Autodesk Inventor part; units mm, degrees
ref_plane "YZ Plane" through (0, 0, 0) normal (1, 0, 0) x (0, 1, 0)
ref_plane "XZ Plane" through (0, 0, 0) normal (0, 1, 0) x (-1, 0, 0)
ref_plane "XY Plane" through (0, 0, 0) normal (0, 0, 1) x (1, 0, 0)
sketch "Sketch1" plane through (0, 0, 0) normal (0, 0, 1) x (1, 0, 0)
  circle A0 centre (0, 0) radius 7.62
  circle A1 centre (0, -40.005) radius 30.48
  circle A2 centre (0, 0) radius 1.55
  circle A3 centre (0, -40.005) radius 1.55
  line L0 (-25.4, 14.478) -> (25.4, 14.478)
  line L1 (25.4, 14.478) -> (25.4, -87.122)
  line L2 (25.4, -87.122) -> (-25.4, -87.122)
  line L3 (-25.4, -87.122) -> (-25.4, 14.478)
  line L4 (-25.4, -87.122) -> (-38.1, -87.122)
  line L5 (-38.1, -87.122) -> (-38.1, -78.232)
  line L6 (-38.1, -78.232) -> (-25.4, -78.232)
  line L7 (25.4, -87.122) -> (38.1, -87.122)
  line L8 (38.1, -87.122) -> (38.1, -78.232)
  line L9 (38.1, -78.232) -> (25.4, -78.232)
  dimension "d0" = 40.005
  dimension "d1" = 15.24
  dimension "d2" = 60.96
  dimension "d3" = 3.1
  dimension "d4" = 3.1
  dimension "d5" = 14.478
  dimension "d6" = 25.4
  dimension "d7" = 25.4
  dimension "d8" = 101.6
  dimension "d9" = 12.7
  dimension "d10" = 12.7
  dimension "d11" = 8.89
extrude "Extrusion1" add sketch "Sketch1" along normal blind 12.7 contours A0 | L1 A1 L3 | A1 L3 L0 L1 | L1 L2 L3 A1 | L9 L8 L7 L1 | L3 L4 L5 L6
sketch "Sketch3" plane through (0, 0, 12.7) normal (0, 0, 1) x (1, 0, 0)
  line L0 (-25.4, -78.232) -> (-38.1, -78.232)
  line L1 (38.1, -87.122) -> (38.1, -78.232)
  line L2 (-38.1, -78.232) -> (38.1, -78.232)
  line L3 (38.1, -78.232) -> (38.1, -87.122)
  line L4 (38.1, -87.122) -> (-38.1, -87.122)
  line L5 (-38.1, -87.122) -> (-38.1, -78.232)
  point P0 (0, 0)
extrude "Extrusion3" add sketch "Sketch3" along normal blind 12.7
sketch "Sketch5" plane through (0, 0, 0) normal (0, 0, -1) x (-1, 0, 0)
  line L0 (38.1, -87.122) -> (-38.1, -87.122)
  line L1 (38.1, -78.232) -> (38.1, -87.122)
  line L2 (-38.1, -87.122) -> (38.1, -87.122)
  line L3 (38.1, -87.122) -> (38.1, -78.232)
  line L4 (38.1, -78.232) -> (-38.1, -78.232)
  line L5 (-38.1, -78.232) -> (-38.1, -87.122)
  point P0 (0, 0)
extrude "Extrusion4" add sketch "Sketch5" along normal blind 4.9022
properties part number "Frame"
For this review, take the finished solid that the model builds, in its own axes (mm). A direction names the side the tool comes from. Give positions to 0.01 mm unless a question says otherwise; leave off trailing zeros. Write each loop counter-clockwise with the first axis right and the second up, starting at its lowest first coordinate (ties: lowest second). Pieces come first, ordered by that corner, then holes. Notation, with made-up numbers: M -22.75,51.5 L 24.25,51.5 A20 ccw 24.25,75.5 Z; hole C 89,-14.75 d11. An arc over 180 degrees is marked long. Answer as a JSON object with one key per item and string values. Group by question number.
Item 1: Tool access review of faces 1 (the flat face through (0, -31, 0)), 2 (the flat face through (0, -31, 12.7)), 3 (the flat face through (-1, -83, 25.4)), 4 (the flat face through (25.4, -31, 6)), 5 (the flat face through (38.1, -83, 10)): name each direction out of +Z, -Z, +X, -X, +Y, -Y from which nothing blocks a thin tool from reaching the whole face with its end or side.
Item 2: For pin 1 Ø10 at (y, z) = (-21.5, 9.5) entering from -X; pin 2 Ø6.5 at (y, z) = (-16, 4) entering from +X; pin 3 Ø1 at (x, y) = (7, -64) entering from +Z; pin 4 Ø2 at (y, z) = (-31.5, 14.5) entering from +X, all flat-tipped, find the tip position at first contact; note any pin that passes through.
Item 3: For probe 1 along Y at (x, z) = (0, 7) (3 decimals); probe 2 along Z at (x, y) = (13, -13.5); probe 3 along X at (y, z) = (-20, 12), list the stretches that pass through material, from the lowest coordinate up. Write a range as [from, to].
Item 4: Consider section B-B on x = 0. Write out the cut boundary in (y, z) (3 decimals).
Item 5: Draft analysis for pull direction X (two halves, no side actions). For faces 6 (the cylindrical face through (-0.336, -38.492, 6.261)), 7 (the cylindrical face through (0.715, 1.375, 6.261)), 8 (the flat face through (-1, -78.232, 14)), 9 (the flat face through (-25.4, -33, 6)), state which applies: +X half, -X half, draft (parallel to the pull), parting line (faces both ways), or undercut.
Item 6: Consider section D-D on x = -28. Write out the cut boundary in (y, z), plus the area to 3 significant figures.
Item 7: Consider section A-A on y = 0. Write out the cut boundary in (x, z).
Item 8: Consider section C-C on z = 6.5. Write out the cut boundary in (x, y) (3 decimals).
Check result:
{
 "1": {"face 1": "-Z, +X, -X, +Y", "face 2": "+Z, +X, -X, +Y", "face 3": "+Z, +X, -X, +Y, -Y", "face 4": "+Z, -Z, +X, +Y", "face 5": "+Z, -Z, +X, +Y, -Y"},
 "2": {"pin 1": "stops at x = -25.4", "pin 2": "stops at x = 25.4", "pin 3": "stops at z = 12.7", "pin 4": "passes through"},
 "3": {"probe 1": "y = [-87.122, -41.555], [-38.455, -1.55], [1.55, 14.478]", "probe 2": "z = [0, 12.7]", "probe 3": "x = [-25.4, 25.4]"},
 "4": {"outline": "M -87.122,-4.902 L -78.232,-4.902 L -78.232,0 L -41.555,0 L -41.555,12.7 L -78.232,12.7 L -78.232,25.4 L -87.122,25.4 Z; M -38.455,0 L -1.55,0 L -1.55,12.7 L -38.455,12.7 Z; M 1.55,0 L 14.478,0 L 14.478,12.7 L 1.55,12.7 Z"},
 "5": {"face 6": "undercut", "face 7": "undercut", "face 8": "draft", "face 9": "-X half"},
 "6": {"outline": "M -87.12,-4.9 L -78.23,-4.9 L -78.23,25.4 L -87.12,25.4 Z", "area": "269 mm^2"},
 "7": {"outline": "M -25.4,0 L -1.55,0 L -1.55,12.7 L -25.4,12.7 Z; M 1.55,0 L 25.4,0 L 25.4,12.7 L 1.55,12.7 Z"},
 "8": {"outline": "M -38.1,-87.122 L 38.1,-87.122 L 38.1,-78.232 L 25.4,-78.232 L 25.4,14.478 L -25.4,14.478 L -25.4,-78.232 L -38.1,-78.232 Z; hole C 0,-40.005 d3.1; hole C 0,0 d3.1"}
}
